Design review of the part built by this model. Coordinates are the model's own, in mm. Round coordinates to 2 decimals unless told otherwise and drop trailing zeros. Write each loop counter-clockwise with the first axis right and the second up, starting at its lowest first coordinate (ties: lowest second). Pieces come first, ordered by that corner, then holes. Notation, with made-up numbers: M 69.5,10 L 97.5,10 A9 cw 97.5,25 Z; hole C -26.5,61.25 d4. An arc over 180 degrees is marked long. One line per question, with ' | ' between items. Start each with the question number.
Item 1: Add section D-D, the plane y = -4. State the section outline as (x, z) points.
Item 2: Insertion check: pin 1 Ø8 at (x, z) = (-50.68, -74) entering from -Y. The pin has a flat end and moves straight along its axis. Give the tip position at first contact, or say it passes through.
Item 3: Add section B-B, the plane x = 25.5. State the section outline as (y, z) points, and give its area (3 significant figures).
Item 4: For L1, parallel to X at y = -4, z = -36; L2, parallel to Z at x = 26.5, y = -5; L3, parallel to Z at x = 45, y = -3.25, list the stretches that pass through material, from the lowest coordinate up.
Item 5: Add section A-A, the plane z = 74. State the section outline as (x, y) points.
Item 6: Add section C-C, the plane z = 23. State the section outline as (x, y) points, and give its area (3 significant figures).
```python
from build123d import *

# Parameters (mm, degrees)
F0_R     = 5
F1_DEPTH = 10
F2_R     = 10
F3_R     = 10


with BuildPart() as f1:
    # F0 (on Front) → F1 (new body)
    with BuildSketch(Plane.XZ):
        with BuildLine():
            Line((-60, -81.5), (60, -81.5))
            Line((60, -81.5), (60, 81.5))
            Line((60, 81.5), (6.165685, 81.5))
            Line((6.165685, 81.5), (6.165685, 52.5))
            Line((6.165685, 52.5), (41, 52.5))
            ThreePointArc((41, 52.5), (48.071068, 49.571068), (51, 42.5))
            Line((51, 42.5), (51, -42.5))
            ThreePointArc((51, -42.5), (48.071068, -49.571068), (41, -52.5))
            Line((41, -52.5), (-41, -52.5))
            ThreePointArc((-41, -52.5), (-48.071068, -49.571068), (-51, -42.5))
            Line((-51, -42.5), (-51, 42.5))
            ThreePointArc((-51, 42.5), (-48.071068, 49.571068), (-41, 52.5))
            Line((-41, 52.5), (-5.834315, 52.5))
            Line((-5.834315, 52.5), (-5.834315, 81.5))
            Line((-5.834315, 81.5), (-60, 81.5))
            Line((-60, 81.5), (-60, -81.5))
        make_face()
        with Locations((-50.680101, -74)):
            Circle(F0_R, mode=Mode.SUBTRACT)
        with Locations((51.650584, -74)):
            Circle(F0_R, mode=Mode.SUBTRACT)
        with Locations((-51.180493, 74)):
            Circle(F0_R, mode=Mode.SUBTRACT)
        with Locations((50.704208, 74)):
            Circle(F0_R, mode=Mode.SUBTRACT)
    extrude(amount=F1_DEPTH)

    # F2
    f2_edges = [f1.edges().sort_by_distance(p)[0] for p in [
        (-5.834315, -5, 52.5),
    ]]
    fillet(f2_edges, radius=F2_R)

    # F3
    f3_edges = [f1.edges().sort_by_distance(p)[0] for p in [
        (6.165685, -5, 52.5),
    ]]
    fillet(f3_edges, radius=F3_R)


solid = f1.part
```
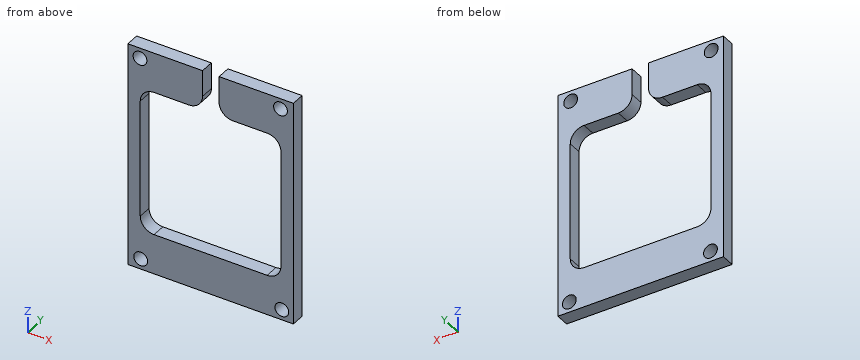
Computed values:
1) outline: M -60,-81.5 L 60,-81.5 L 60,81.5 L 6.17,81.5 L 6.17,62.5 A10 ccw 16.17,52.5 L 41,52.5 A10 cw 51,42.5 L 51,-42.5 A10 cw 41,-52.5 L -41,-52.5 A10 cw -51,-42.5 L -51,42.5 A10 cw -41,52.5 L -15.83,52.5 A10 ccw -5.83,62.5 L -5.83,81.5 L -60,81.5 Z; hole C -51.18,74 d10; hole C -50.68,-74 d10; hole C 50.7,74 d10; hole C 51.65,-74 d10
2) pin 1: passes through
3) outline: M -10,-81.5 L 0,-81.5 L 0,-52.5 L -10,-52.5 Z; M -10,52.5 L 0,52.5 L 0,81.5 L -10,81.5 Z | area: 580 mm^2
4) L1: x = -60 to -51, 51 to 60 | L2: z = -81.5 to -52.5, 52.5 to 81.5 | L3: z = -81.5 to -51.67, 51.67 to 81.5
5) outline: M -60,-10 L -56.18,-10 L -56.18,0 L -60,0 Z; M -46.18,-10 L -5.83,-10 L -5.83,0 L -46.18,0 Z; M 6.17,-10 L 45.7,-10 L 45.7,0 L 6.17,0 Z; M 55.7,-10 L 60,-10 L 60,0 L 55.7,0 Z
6) outline: M -60,-10 L -51,-10 L -51,0 L -60,0 Z; M 51,-10 L 60,-10 L 60,0 L 51,0 Z | area: 180 mm^2
